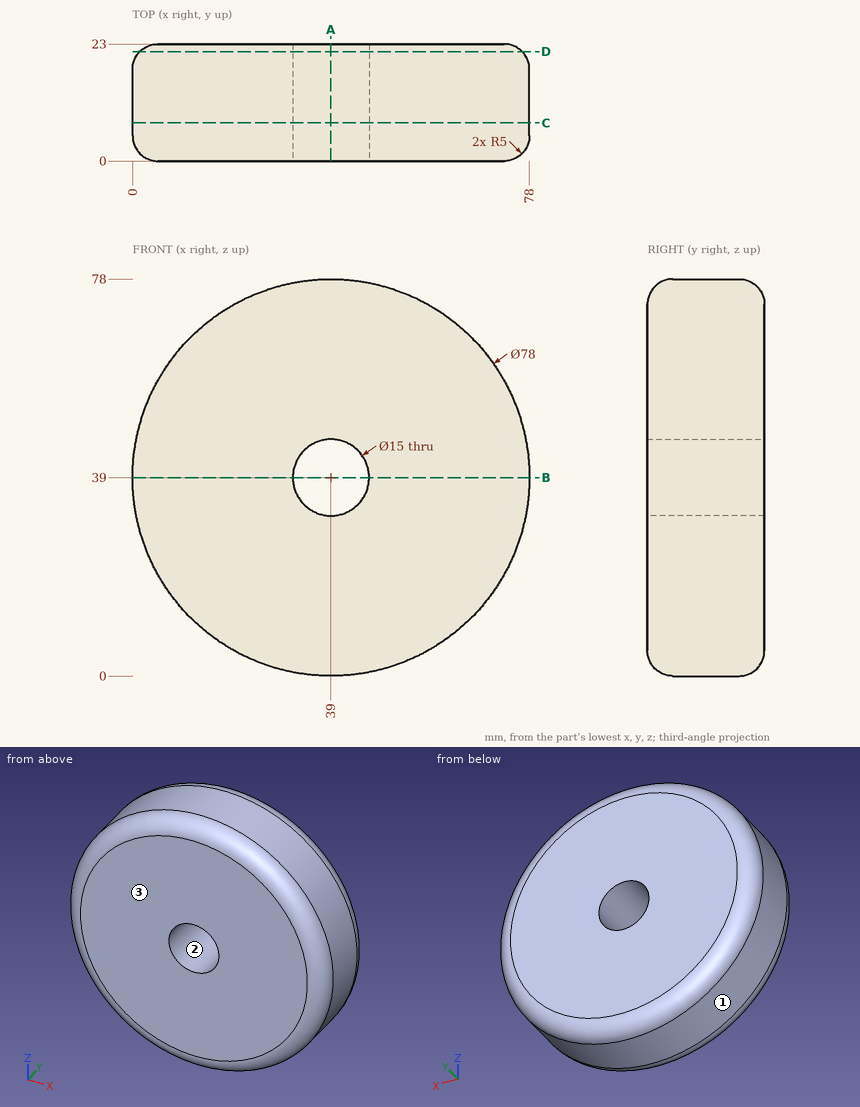
Source: three-view drawing plus pictorial views. Frame: mm from the lowest corner of the part. Round coordinates to 2 decimals unless told otherwise and drop trailing zeros. Order: outer loops, then holes, each group sorted by start corner. A loop starts at its lowest first (then second) coordinate and runs counter-clockwise, first axis right, second up. Notation, with made-up numbers: (-10.75, 56) - (46.25, 56) arc R20 cw to (46.25, 85) - close; hole circle Ø10 at (-12, 76.5). An arc over 180 degrees is marked (long way). Write each question's results on one line, items separated by ' | '.
Item 1: Section C-C, the plane y = 7.5. Return the cut outline in (x, z).
Completed:
outline: circle Ø78 at (39, 39); hole circle Ø15 at (39, 39)
Item 2: Mould query, pull axis X, two halves, no side actions, for the marked faces 1, 2 and 3. Classes: pulls with the +X half, pulls with the -X half, needs draft (parallel to the pull), parting line crosses it, or undercut.
Completed:
face 1: parting line crosses it | face 2: undercut | face 3: needs draft
Item 3: Section D-D, the plane y = 21.5. Return the cut outline in (x, z), and give its area (3 significant figures).
Completed:
outline: circle Ø75.14 at (39, 39); hole circle Ø15 at (39, 39) | area: 4,260 mm^2
Item 4: Section B-B, the plane z = 39. Return the cut outline in (x, y), and give its area (3 significant figures).
Completed:
outline: (0, 5) arc R5 ccw to (5, 0) - (31.5, 0) - (31.5, 23) - (5, 23) arc R5 ccw to (0, 18) - close; (46.5, 0) - (73, 0) arc R5 ccw to (78, 5) - (78, 18) arc R5 ccw to (73, 23) - (46.5, 23) - close | area: 1,430 mm^2
Item 5: Section A-A, the plane x = 39. Return the cut outline in (y, z), and give its area (3 significant figures).
Completed:
outline: (0, 5) arc R5 ccw to (5, 0) - (18, 0) arc R5 ccw to (23, 5) - (23, 31.5) - (0, 31.5) - close; (0, 46.5) - (23, 46.5) - (23, 73) arc R5 ccw to (18, 78) - (5, 78) arc R5 ccw to (0, 73) - close | area: 1,430 mm^2
Item 6: First-contact query: pin 1 Ø1.5 at (x, y) = (69, 4) entering from -Z; pin 2 Ø1 at (y, z) = (7.5, 39) entering from +X; pin 3 Ø9 at (x, z) = (39, 39) entering from -Y; pin 4 Ø1 at (y, z) = (17.5, 35.5) entering from +X. Flat tips, straight axial feed; report the tip coordinate or a pass-through.
Completed:
pin 1: z = 13.33 | pin 2: x = 78 | pin 3: through | pin 4: x = 77.88
Item 7: Material intervals for line 1 along X through (y, z) = (9.75, 39); line 2 along X through (y, z) = (18.5, 44); line 3 along Z through (x, y) = (41.5, 6), sorted ascending. Write a range as [from, to].
Completed:
line 1: [0, 31.5], [46.5, 78] | line 2: [0.35, 33.41], [44.59, 77.65] | line 3: [0.08, 31.93], [46.07, 77.92]
